from build123d import *

# Parameters (mm, degrees)
SKETCH_W   = 600
SKETCH_H   = 300
SKETCH_R   = 12
SKETCH_W_2 = 28
SKETCH_H_2 = 48
PAD_DEPTH  = 15


with BuildPart() as part:
    # Sketch → Pad (new body)
    with BuildSketch(Plane.YZ):
        with Locations((300, 150)):
            Rectangle(SKETCH_W, SKETCH_H)
        with Locations((200, 40)):
            Circle(SKETCH_R, mode=Mode.SUBTRACT)
        with Locations((266.666667, 40)):
            Circle(SKETCH_R, mode=Mode.SUBTRACT)
        with Locations((333.333333, 40)):
            Circle(SKETCH_R, mode=Mode.SUBTRACT)
        with Locations((400, 40)):
            Circle(SKETCH_R, mode=Mode.SUBTRACT)
        with Locations((54, 150)):
            Rectangle(SKETCH_W_2, SKETCH_H_2, mode=Mode.SUBTRACT)
    extrude(amount=PAD_DEPTH)


solid = part.part
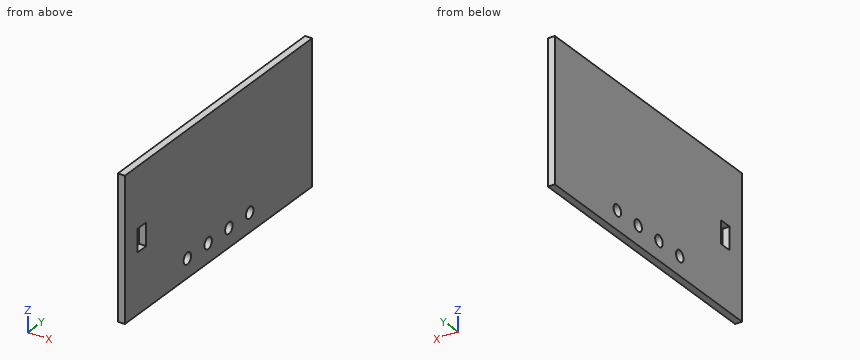
Geometry: final body of the model. Coordinates: model frame, mm. Round coordinates to 2 decimals unless told otherwise and drop trailing zeros. Loops run counter-clockwise (first coordinate to the right, second up) from the corner with the lowest first, then second, coordinate; pieces in that order, holes last. Notation, with made-up numbers: (68.25, 73) - (104.25, 73) arc R11 ccw to (104.25, 92) - close; hole circle Ø3 at (89, -15.75). An arc over 180 degrees is marked (long way). Write each question's results on one line, items separated by ' | '. Start each with the question number.
1) Cut plane A-A on z = 40. Return loops of the section in (x, y), then the cut area to 3 significant figures.
2) Cut plane D-D on x = 9.25. Return loops of the section in (y, z).
3) Cut plane C-C on z = 161. Return loops of the section in (x, y), then the cut area to 3 significant figures.
4) Line query: probe 1 along Z at (x, y) = (13.25, 341); probe 2 along Z at (x, y) = (10.5, 192.5). Output: solid intervals per line, ascending. Write a range as [from, to].
5) Cut plane B-B on y = 400. Return loops of the section in (x, z), then the cut area to 3 significant figures.
Verdict:
1) outline: (0, 0) - (15, 0) - (15, 188) - (0, 188) - close; (0, 212) - (15, 212) - (15, 254.67) - (0, 254.67) - close; (0, 278.67) - (15, 278.67) - (15, 321.33) - (0, 321.33) - close; (0, 345.33) - (15, 345.33) - (15, 388) - (0, 388) - close; (0, 412) - (15, 412) - (15, 600) - (0, 600) - close | area: 7,560 mm2
2) outline: (0, 0) - (600, 0) - (600, 300) - (0, 300) - close; hole (40, 126) - (68, 126) - (68, 174) - (40, 174) - close; hole circle Ø24 at (200, 40); hole circle Ø24 at (266.67, 40); hole circle Ø24 at (333.33, 40); hole circle Ø24 at (400, 40)
3) outline: (0, 0) - (15, 0) - (15, 40) - (0, 40) - close; (0, 68) - (15, 68) - (15, 600) - (0, 600) - close | area: 8,580 mm2
4) probe 1: z = [0, 30.77], [49.23, 300] | probe 2: z = [0, 30.63], [49.37, 300]
5) outline: (0, 0) - (15, 0) - (15, 28) - (0, 28) - close; (0, 52) - (15, 52) - (15, 300) - (0, 300) - close | area: 4,140 mm2
